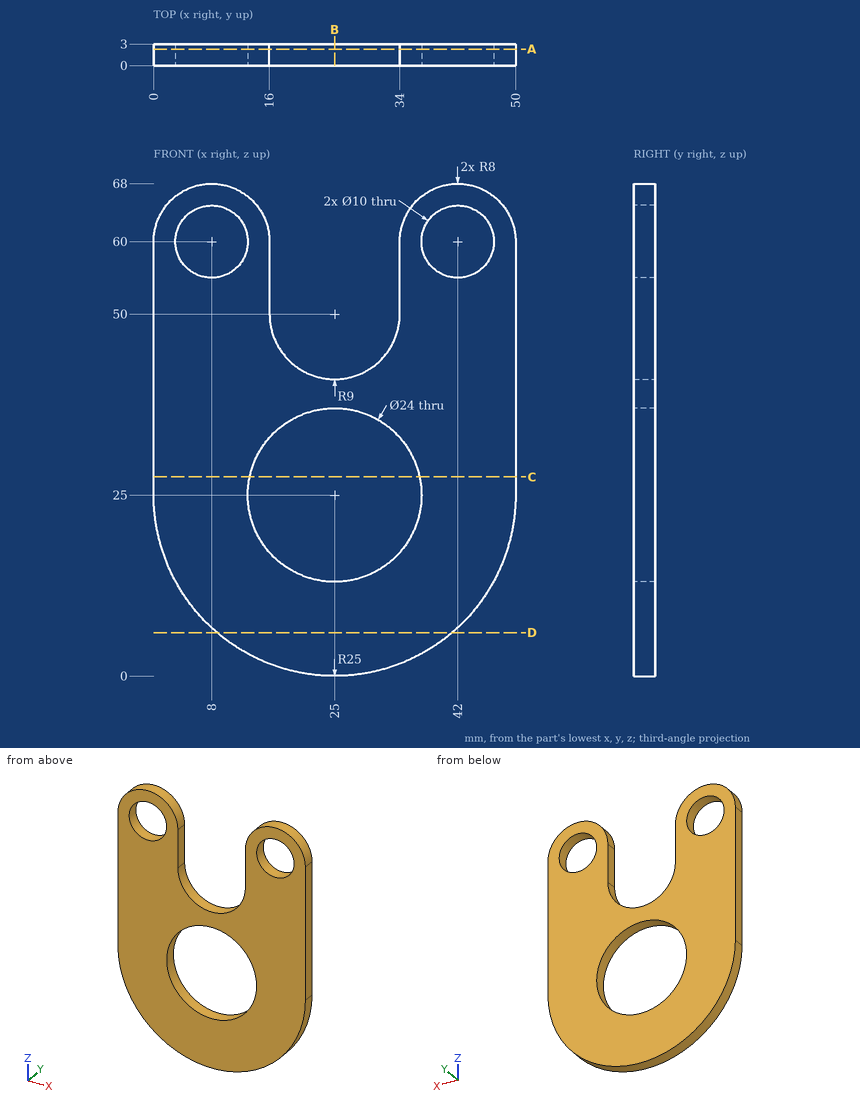
The figure shows three views and two pictorial views of one solid part (mm, origin at its lowest corner). Answer the questions. Coordinates: 2 decimals unless noted, no trailing zeros. Loops run counter-clockwise (first coordinate to the right, second up) from the corner with the lowest first, then second, coordinate; pieces in that order, holes last. Notation, with made-up numbers: (20.25, -35) -> (53.25, -35) arc R20 cw to (53.25, -12) -> close; hole circle Ø3 at (44.25, 68). An arc over 180 degrees is marked (long way). Return JSON: item names as keys, results as strings. Group by question number.
(1) A cutting plane is placed at C-C on z = 27.5. Write down the section's boundary in (x, y), and give its area (3 significant figures).
(2) Given pin 1 Ø1.5 at (y, z) = (1.5, 8) entering from -X, flat-ended and moving along its own axis, determine where the tip first touches the part or whether it passes through.
(3) A cutting plane is placed at B-B on x = 25. Write down the section's boundary in (y, z), and give its area (3 significant figures).
(4) A cutting plane is placed at A-A on y = 2.3. Write down the section's boundary in (x, z), and give its area (3 significant figures).
(5) Find the intervals of material crossed by probe 1 along X at (y, z) = (1.2, 25); probe 2 along X at (y, z) = (0.65, 60); probe 3 along X at (y, z) = (2.55, 56.5), in increasing order. Write a range as from..to.
(6) A cutting plane is placed at D-D on z = 6. Write down the section's boundary in (x, y), and give its area (3 significant figures).
The answers:
{
 "1": {"outline": "(0, 0) -> (13.26, 0) -> (13.26, 3) -> (0, 3) -> close; (36.74, 0) -> (50, 0) -> (50, 3) -> (36.74, 3) -> close", "area": "79.6 mm^2"},
 "2": {"pin 1": "stops at x = 6"},
 "3": {"outline": "(0, 0) -> (3, 0) -> (3, 13) -> (0, 13) -> close; (0, 37) -> (3, 37) -> (3, 41) -> (0, 41) -> close", "area": "51.0 mm^2"},
 "4": {"outline": "(0, 25) arc R25 ccw to (50, 25) -> (50, 60) arc R8 ccw to (34, 60) -> (34, 50) arc R9 cw to (16, 50) -> (16, 60) arc R8 ccw to (0, 60) -> close; hole circle Ø10 at (8, 60); hole circle Ø24 at (25, 25); hole circle Ø10 at (42, 60)", "area": "2,020 mm^2"},
 "5": {"probe 1": "x = 0..13, 37..50", "probe 2": "x = 0..3, 13..16, 34..37, 47..50", "probe 3": "x = 0..4.43, 11.57..16, 34..38.43, 45.57..50"},
 "6": {"outline": "(8.75, 0) -> (41.25, 0) -> (41.25, 3) -> (8.75, 3) -> close", "area": "97.5 mm^2"}
}
